Autodesk Inventor part; units mm, degrees
ref_plane "YZ Plane" through (0, 0, 0) normal (1, 0, 0) x (0, 1, 0)
ref_plane "XZ Plane" through (0, 0, 0) normal (0, 1, 0) x (-1, 0, 0)
ref_plane "XY Plane" through (0, 0, 0) normal (0, 0, 1) x (1, 0, 0)
sketch "Sketch1" plane through (0, 0, 0) normal (0, 0, 1) x (1, 0, 0)
  line L0 (0, 0) -> (0, 14.351)
  line L1 (0, 0) -> (14.351, 0) construction
  line L2 (0, 14.351) -> (16.51, 14.351)
  line L3 (16.51, 14.351) -> (16.51, 27.051)
  line L4 (16.51, 27.051) -> (34.29, 27.051)
  line L5 (34.29, 27.051) -> (34.29, 12.7)
  line L6 (34.29, 12.7) -> (12.7, 12.7)
  line L7 (12.7, 12.7) -> (12.7, 0)
  line L8 (0, 0) -> (12.7, 0)
  dimension "d0" = 14.351
  dimension "d2" = 16.51
  dimension "d6" = 17.78
  dimension "d9" = 21.59
  dimension "d47" = 14.351
  dimension "d49" = 12.7
extrude "Extrusion1" add sketch "Sketch1" along normal blind 127
sketch "Sketch3" plane through (16.51, 27.051, 0) normal (0, 1, 0) x (1, 0, 0)
  line L0 (0, -127) -> (-16.51, -127)
  line L1 (-16.51, 0) -> (0, 0)
  line L2 (-16.51, 0) -> (-16.51, -127)
  point P0 (-10.16, -12.7)
  point P1 (-10.16, -114.3)
  dimension "d25" = 12.7
  dimension "d26" = 12.7
  dimension "d27" = 6.35
  dimension "d28" = 6.35
hole "Hole2" at (6.35, 27.051, 12.7) at (6.35, 27.051, 114.3) direction (0, -1, 0) diameter 6.35 end through all
sketch "Sketch4" plane through (16.51, 27.051, 0) normal (0, 1, 0) x (1, 0, 0)
  line L0 (17.78, 0) -> (17.78, -127)
  line L1 (17.78, -127) -> (0, -127)
  line L2 (0, 0) -> (17.78, 0)
  line L3 (0, 0) -> (0, -127)
  point P0 (-16.51, 0)
  point P1 (8.89, -12.7)
  point P2 (8.89, -114.3)
  dimension "d36" = 8.89
  dimension "d37" = 12.7
  dimension "d38" = 12.7
  dimension "d48" = 17.78
hole "Hole3" at (25.4, 27.051, 12.7) at (25.4, 27.051, 114.3) direction (0, -1, 0) diameter 6.35 end through all
chamfer "Chamfer1" distance 3.556 angle 45 2 edges at (16.51, 14.351, 63.5) (12.7, 12.7, 63.5)
chamfer "Chamfer2" distance 2.54 angle 45 2 edges at (34.29, 12.7, 63.5) (16.51, 27.051, 63.5)
equation "\"d0\" = d47"
properties part number "Block_3-8" material "Aluminum 6061"
Can you work these out from the model? Positions are in its coordinate system, mm. A direction names the side the tool comes from. Round coordinates to 2 decimals unless told otherwise and drop trailing zeros. Order: outer loops, then holes, each group sorted by start corner. A loop starts at its lowest first (then second) coordinate and runs counter-clockwise, first axis right, second up. Notation, with made-up numbers: M 9.5,-9 L 21.5,-9 A10 cw 21.5,-5 Z; hole C 79,29.5 d4. An arc over 180 degrees is marked long. Use a Markdown table: item, result.
1) On a 3-axis mill with a long thin cutter (end or side, diameter ignored), from which of +Z, -Z, +X, -X, +Y, -Y can I reach the whole of each face in a straight line? I mean faces 5 (the face through (24, 12.7, 63)), 6 (the face through (17, 14, 0)). Say none if no direction works.
Geometry says:
| item | result |
|---|---|
| face 5 | +Z, -Z, +X, -Y |
| face 6 | -Z, +X, -X, +Y, -Y |
2) If we mould it in two halves opening along X, with no side actions, what happens to faces 1 (the face through (14.503, 10.947, 62.611)), 2 (the face through (23.254, 19.775, 10.36)), 3 (the face through (6, 14.351, 63)), 4 (the face through (16.51, 21, 63))? For each: +X half, -X half, draft (parallel to the pull), parting line (faces both ways), or undercut.
Geometry says:
| item | result |
|---|---|
| face 1 | +X half |
| face 2 | undercut |
| face 3 | draft |
| face 4 | -X half |
3) Imagine slicing it at A-A (x = 25.4). List the corners of the cut face in (y, z) for me (3 decimals).
Geometry says:
| item | result |
|---|---|
| outline | M 12.7,0 L 27.051,0 L 27.051,9.525 L 12.7,9.525 Z; M 12.7,15.875 L 27.051,15.875 L 27.051,111.125 L 12.7,111.125 Z; M 12.7,117.475 L 27.051,117.475 L 27.051,127 L 12.7,127 Z |
4) Imagine slicing it at D-D (z = 82). List the corners of the cut face in (x, y) for me.
Geometry says:
| item | result |
|---|---|
| outline | M 0,0 L 12.7,0 L 12.7,9.14 L 16.26,12.7 L 31.75,12.7 L 34.29,15.24 L 34.29,27.05 L 19.05,27.05 L 16.51,24.51 L 16.51,17.91 L 12.95,14.35 L 0,14.35 Z |
5) If I drill on line 1 along Z through (x, y) = (25.4, 20.5) (3 decimals); line 2 along X through (y, z) = (23.75, 12.7) (3 decimals); line 3 along Z through (x, y) = (9, 12), over which ranges is the centre line in solid material (lowest first)?
Geometry says:
| item | result |
|---|---|
| line 1 | z = 0 to 9.525, 15.875 to 111.125, 117.475 to 127 |
| line 2 | x = 16.51 to 22.225, 28.575 to 34.29 |
| line 3 | z = 0 to 10.95, 14.45 to 112.55, 116.05 to 127 |
6) Imagine slicing it at C-C (y = 20.5). List the corners of the cut face in (x, z) for me (3 decimals), then the cut area to 3 significant figures.
Geometry says:
| item | result |
|---|---|
| outline | M 16.51,0 L 34.29,0 L 34.29,127 L 16.51,127 Z; hole C 25.4,12.7 d6.35; hole C 25.4,114.3 d6.35 |
| area | 2,190 mm² |
7) I'm going to push flat-ended pins straight in: P1, Ø4, axis at x = 9.5, z = 39.5, coming from the +Y side; P2, Ø17, axis at x = 24, z = 77, coming from the -Y side; P3, Ø7.5, axis at x = 25.4, z = 114.3, coming from the -Y side. Where does each tip first touch, or does it pass through?
Geometry says:
| item | result |
|---|---|
| P1 | stops at y = 14.35 |
| P2 | stops at y = 11.94 |
| P3 | stops at y = 12.7 |
8) Imagine slicing it at B-B (z = 114.3). List the corners of the cut face in (x, y) for me (3 decimals), then the cut area to 3 significant figures.
Geometry says:
| item | result |
|---|---|
| outline | M 0,0 L 3.175,0 L 3.175,14.351 L 0,14.351 Z; M 9.525,0 L 12.7,0 L 12.7,9.144 L 16.256,12.7 L 22.225,12.7 L 22.225,27.051 L 19.05,27.051 L 16.51,24.511 L 16.51,17.907 L 12.954,14.351 L 9.525,14.351 Z; M 28.575,12.7 L 31.75,12.7 L 34.29,15.24 L 34.29,27.051 L 28.575,27.051 Z |
| area | 268 mm² |
